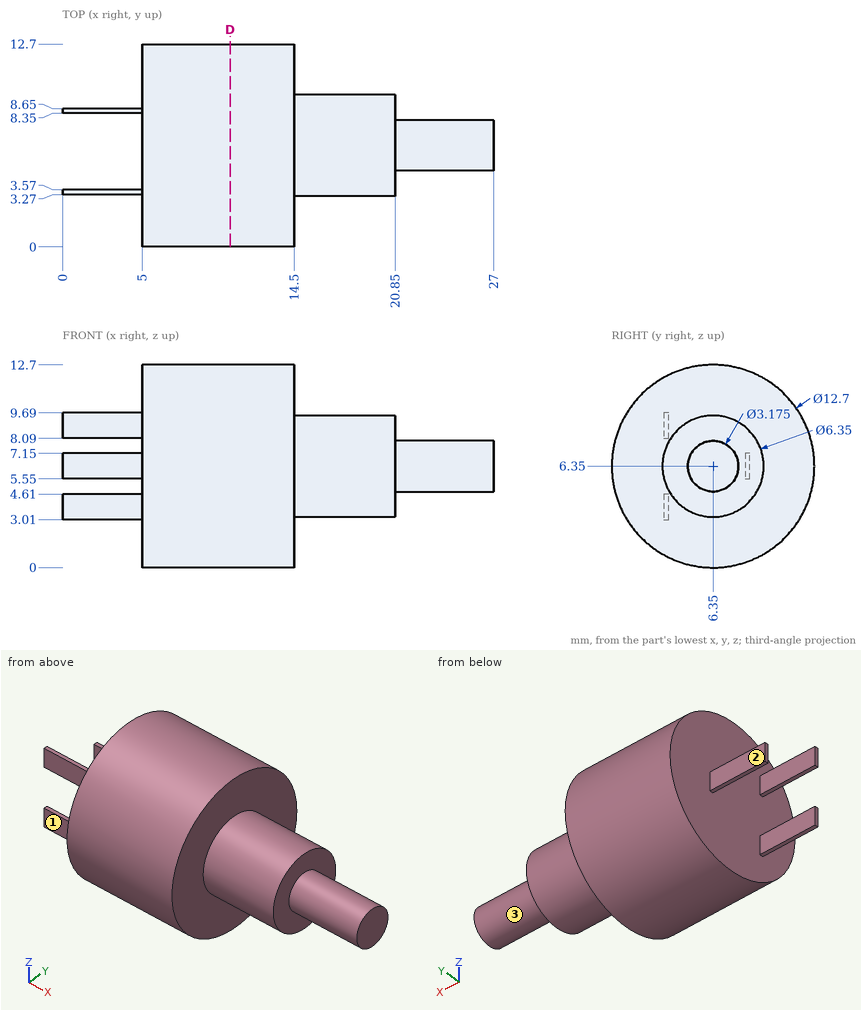
For this review, use the dimensioned drawing (mm, ordinates from the lowest corner) and the shaded views. A direction names the side the tool comes from. Round coordinates to 2 decimals unless told otherwise and drop trailing zeros. Order: outer loops, then holes, each group sorted by start corner. A loop starts at its lowest first (then second) coordinate and runs counter-clockwise, first axis right, second up. Notation, with made-up numbers: M 81.25,81.25 L 120.25,81.25 A17 ccw 120.25,92.25 Z; hole C 30,37 d5. An arc over 180 degrees is marked long. Use a Markdown table: item, result.
1) Insertion check: pin 1 (0.5 mm diameter, centred on x = 2.5, z = 6.5, fed in from +Y); pin 2 (1.8 mm diameter, centred on x = 3, z = 6, fed in from -Y); pin 3 (5 mm diameter, centred on x = 18.5, y = 8.5, fed in from -Z) (3 decimals); pin 4 (4 mm diameter, centred on y = 4.5, z = 9, fed in from +X). Each pin has a flat end and moves straight along its axis. Give the tip position at first contact, or say it passes through.
Report:
| item | result |
|---|---|
| pin 1 | y = 8.65 |
| pin 2 | y = 8.35 |
| pin 3 | z = 3.175 |
| pin 4 | x = 27 |
2) Wall thickness on line 1 along X through (y, z) = (4, 2); line 2 along X through (y, z) = (8, 4.5); line 3 along Y through (x, z) = (24.5, 5): over which ranges is each line inside the solid? List them lowest first. Write a range as [from, to].
Report:
| item | result |
|---|---|
| line 1 | [5, 14.5] |
| line 2 | [5, 20.85] |
| line 3 | [5.51, 7.19] |
3) Consider section D-D (x = 10.5). Write out the cut boundary in (y, z), then the cut area to 3 significant figures.
Report:
| item | result |
|---|---|
| outline | C 6.35,6.35 d12.7 |
| area | 127 mm^2 |
4) Tool access review of the marked faces 1, 2 and 3: name each direction out of +Z, -Z, +X, -X, +Y, -Y from which nothing blocks a thin tool from reaching the whole face with its end or side.
Report:
| item | result |
|---|---|
| face 1 | +Z, -Z, -X, -Y |
| face 2 | +Z, -Z, -X, +Y |
| face 3 | +X |
